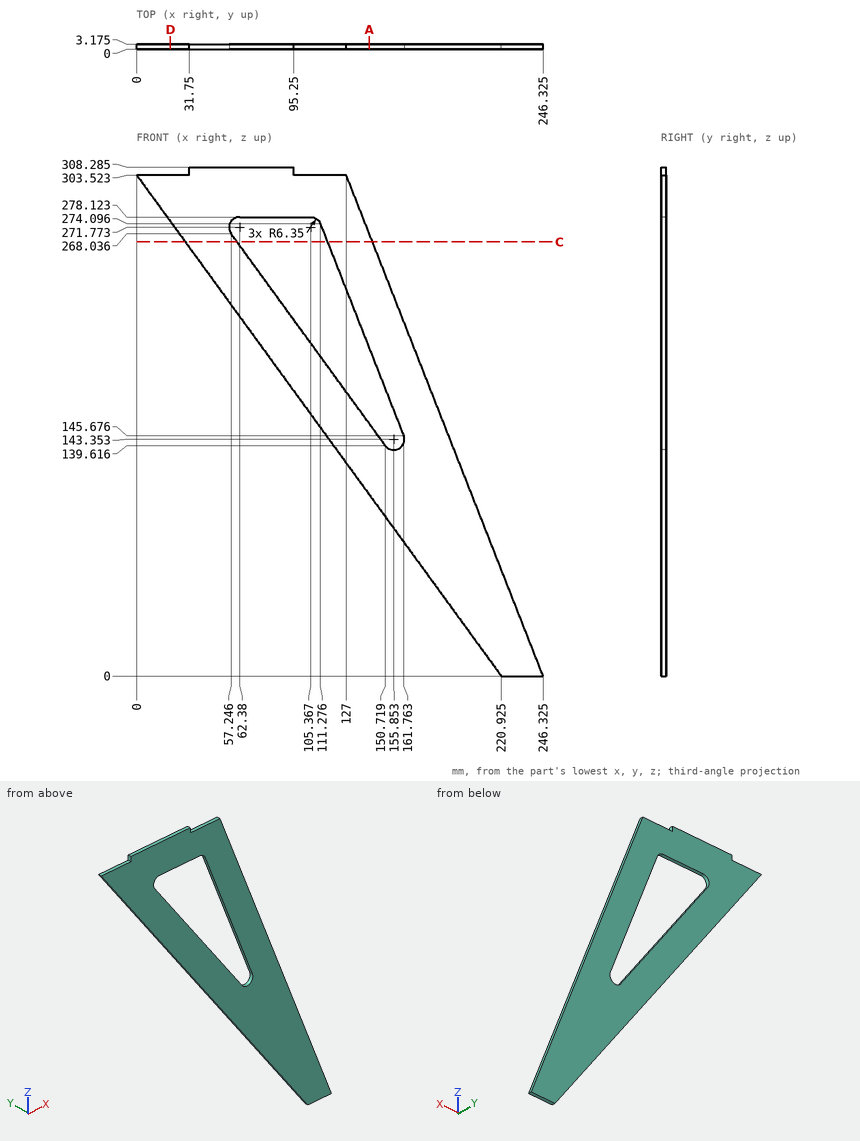
Geometry: see drawing. Coordinates: mm, zero at the bounding-box minimum. Give positions to 0.01 mm unless a question says otherwise; leave off trailing zeros. Order: outer loops, then holes, each group sorted by start corner. A loop starts at its lowest first (then second) coordinate and runs counter-clockwise, first axis right, second up.
Q1. Ray query, probe 1 along Z at (x, y) = (57, 2.85) (1 decimal); probe 2 along Z at (x, y) = (104.5, 0.35) (1 decimal); probe 3 along X at (y, z) = (2.65, 48.5) (1 decimal). Return the intervals inside material, ascending.
Checked values:
probe 1: z = 225.2 to 268.4, 275.1 to 308.3
probe 2: z = 160 to 203.1, 278.1 to 303.5
probe 3: x = 185.6 to 227.3
Q2. Contact query for flat-ended pins moving along their axis: pin 1 Ø1.6 at (x, y) = (106, 2) entering from +Z; pin 2 Ø1 at (y, z) = (2, 176.5) entering from -X; pin 3 Ø1 at (y, z) = (2, 305.5) entering from -X. Output: stop coordinate, or through.
Checked values:
pin 1: stops at z = 303.52
pin 2: stops at x = 92.09
pin 3: stops at x = 31.75
Q3. Section D-D on x = 20.5. Output: boundary loops of the cut face in (y, z) (1 decimal).
Checked values:
outline: (0, 275.4) - (3.2, 275.4) - (3.2, 303.5) - (0, 303.5) - close
Q4. Section C-C on z = 263. Output: boundary loops of the cut face in (x, y) (1 decimal).
Checked values:
outline: (29.5, 0) - (60.9, 0) - (60.9, 3.2) - (29.5, 3.2) - close; (115.6, 0) - (142.9, 0) - (142.9, 3.2) - (115.6, 3.2) - close
Q5. Section A-A on x = 141. Output: boundary loops of the cut face in (y, z) (1 decimal).
Checked values:
outline: (0, 109.8) - (3.2, 109.8) - (3.2, 153) - (0, 153) - close; (0, 198.5) - (3.2, 198.5) - (3.2, 267.9) - (0, 267.9) - close
